Here's the drawing with two shaded views (mm, measured from the low corner). I have some questions. Coordinates: 2 decimals unless noted, no trailing zeros. Loops run counter-clockwise (first coordinate to the right, second up) from the corner with the lowest first, then second, coordinate; pieces in that order, holes last. Notation, with made-up numbers: (-4, -8) - (47, -8) arc R26 cw to (47, 27) - close; hole circle Ø3 at (49.5, 24). An arc over 180 degrees is marked (long way). One line per item, written item: value. Start each with the question number.
(1) If we section it at A-A on y = 4.25: Write out the boundary of the cut face in (x, z), then the cut area to 3 significant figures.
(2) If we section it at D-D on z = 6.5: Write out the boundary of the cut face in (x, y).
(3) If we section it at C-C on x = 4.75: Write out the boundary of the cut face in (y, z), then the cut area to 3 significant figures.
(4) If I drill on line 1 along X through (y, z) = (2, 6.25); line 2 along X through (y, z) = (3.75, 4.5); line 3 along Y through (x, z) = (23.75, 3.5), over which ranges is the centre line in solid material (lowest first)? Write a range as from..to.
(5) I'm going to push flat-ended pins straight in: P1, Ø4, axis at y = 1.5, z = 6, coming from the -X side; P2, Ø5, axis at x = 10.5, z = 7.5, coming from the -Y side; P3, Ø3, axis at x = 15.5, y = 2, coming from the +Z side. Where does each tip first touch, or does it pass through?
(6) If we section it at B-B on z = 4.25: Write out the boundary of the cut face in (x, y).
(7) If we mould it in two halves opening along X, with no side actions, what happens to the marked faces 1, 2 and 3? For each: pulls with the +X half, pulls with the -X half, needs draft (parallel to the pull), parting line crosses it, or undercut.
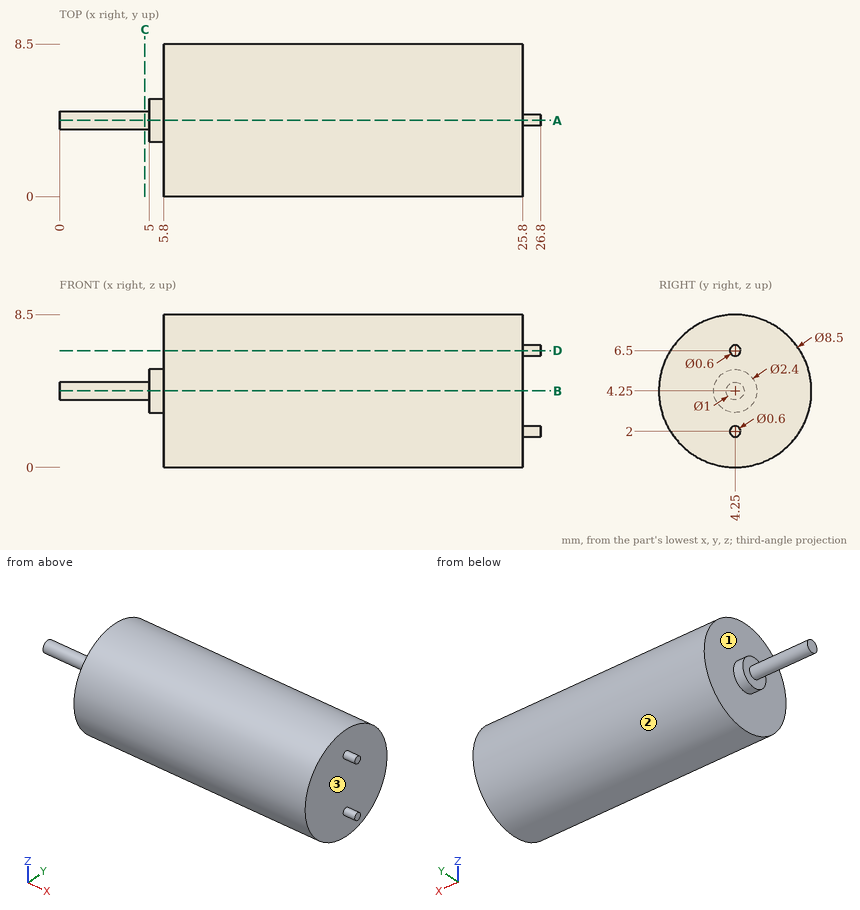
Values:
1. outline: (0, 3.75) - (5, 3.75) - (5, 3.05) - (5.8, 3.05) - (5.8, 0) - (25.8, 0) - (25.8, 1.7) - (26.8, 1.7) - (26.8, 2.3) - (25.8, 2.3) - (25.8, 6.2) - (26.8, 6.2) - (26.8, 6.8) - (25.8, 6.8) - (25.8, 8.5) - (5.8, 8.5) - (5.8, 5.45) - (5, 5.45) - (5, 4.75) - (0, 4.75) - close
1. area: 178 mm2
2. outline: (5.8, 0.64) - (25.8, 0.64) - (25.8, 3.95) - (26.8, 3.95) - (26.8, 4.55) - (25.8, 4.55) - (25.8, 7.86) - (5.8, 7.86) - close
3. outline: circle Ø1 at (4.25, 4.25)
3. area: 0.785 mm2
4. line 1: x = 5.8..25.8
4. line 2: x = 5..25.8
4. line 3: y = 0.07..8.43
5. P1: stops at x = 5.8
5. P2: stops at y = 0.07
5. P3: stops at z = 8.43
6. outline: (0, 3.75) - (5, 3.75) - (5, 3.05) - (5.8, 3.05) - (5.8, 0) - (25.8, 0) - (25.8, 8.5) - (5.8, 8.5) - (5.8, 5.45) - (5, 5.45) - (5, 4.75) - (0, 4.75) - close
7. face 1: pulls with the -X half
7. face 2: needs draft
7. face 3: pulls with the +X half
